Verification items for this drawing (mm, ordinates from the low corner). A direction names the side the tool comes from. Coordinates: 2 decimals unless noted, no trailing zeros. Order: outer loops, then holes, each group sorted by start corner. A loop starts at its lowest first (then second) coordinate and runs counter-clockwise, first axis right, second up. Notation, with made-up numbers: M 28.5,-11 L 68.5,-11 A17 cw 68.5,-2 Z; hole C -34.5,50.5 d1. An arc over 180 degrees is marked long. Return JSON: item names as keys, results as strings. Group by question number.
1. Section check B-B, the plane x = 6. Record the cut outline in (y, z).
2. Set-up check for the marked faces 1, 2 and 3: record each of +Z, -Z, +X, -X, +Y, -Y from which the full face is reachable in a straight line by a thin tool's end or side.
3. Gauge pin test, flat end, axial feed: pin 1 (4 mm diameter, centred on x = 8.5, y = 19, fed in from +Z). Record the tip position at first contact, or that the pin passes through.
4. Section check D-D, the plane z = 23.75. Record the cut outline in (x, y).
5. Mould release check, pull along Y, two halves, no side actions. Record for the marked faces 4, 5 and 6: +Y half, -Y half, draft (parallel to the pull), parting line (faces both ways), or undercut.
6. Section check C-C, the plane y = 51. Record the cut outline in (x, z), plus the area to 3 significant figures.
7. Section check A-A, the plane z = 4. Record the cut outline in (x, y).
8. Material ranges on line 1 along Y through (x, z) = (3.25, 6.75); line 2 along Z through (x, y) = (12, 38); line 3 along Y through (x, z) = (2.25, 18.75), recorded low to high.
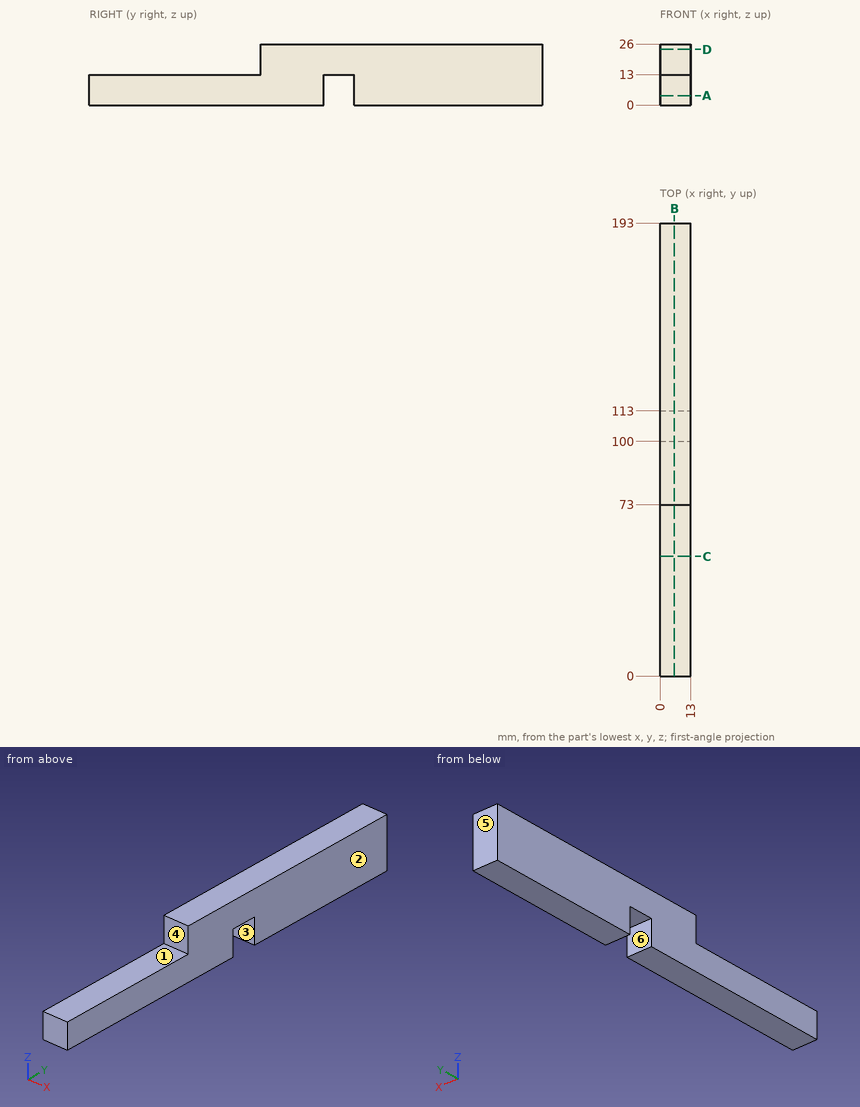
Answers follow:
{
 "1": {"outline": "M 0,0 L 100,0 L 100,13 L 113,13 L 113,0 L 193,0 L 193,26 L 73,26 L 73,13 L 0,13 Z"},
 "2": {"face 1": "+Z, +X, -X, -Y", "face 2": "+Z, -Z, +X, +Y, -Y", "face 3": "-Z, +X, -X"},
 "3": {"pin 1": "z = 13"},
 "4": {"outline": "M 0,73 L 13,73 L 13,193 L 0,193 Z"},
 "5": {"face 4": "-Y half", "face 5": "+Y half", "face 6": "undercut"},
 "6": {"outline": "M 0,0 L 13,0 L 13,13 L 0,13 Z", "area": "169 mm^2"},
 "7": {"outline": "M 0,0 L 13,0 L 13,100 L 0,100 Z; M 0,113 L 13,113 L 13,193 L 0,193 Z"},
 "8": {"line 1": "0 to 100, 113 to 193", "line 2": "0 to 13", "line 3": "73 to 193"}
}
